from build123d import *

# Parameters (mm, degrees)
SKETCH1_R           = 4
SKETCH1_R_2         = 12
BOSS_EXTRUDE1_DEPTH = 5
CUT_EXTRUDE1_REACH  = 55.898
CHAMFER1_SIZE       = 1


with BuildPart() as part:
    # Sketch1 → Boss-Extrude1 (new body)
    with BuildSketch(Plane.XY):
        with BuildLine():
            Line((-40.864864865, 10.298680477), (-8.432432432, 22.469848314))
            ThreePointArc((-8.432432432, 22.469848314), (0, 24), (8.432432432, 22.469848314))
            Line((8.432432432, 22.469848314), (40.864864865, 10.298680477))
            ThreePointArc((40.864864865, 10.298680477), (48, 0), (40.864864865, -10.298680477))
            Line((40.864864865, -10.298680477), (8.432432432, -22.469848314))
            ThreePointArc((8.432432432, -22.469848314), (0, -24), (-8.432432432, -22.469848314))
            Line((-8.432432432, -22.469848314), (-40.864864865, -10.298680477))
            ThreePointArc((-40.864864865, -10.298680477), (-48, 0), (-40.864864865, 10.298680477))
        make_face()
        with Locations((-37, 0)):
            Circle(SKETCH1_R, mode=Mode.SUBTRACT)
        with Locations((37, 0)):
            Circle(SKETCH1_R, mode=Mode.SUBTRACT)
        Circle(SKETCH1_R_2, mode=Mode.SUBTRACT)
    extrude(amount=BOSS_EXTRUDE1_DEPTH)

    # Sketch2 → Cut-Extrude1 (cut, up to next)
    with BuildSketch(Plane.XY.offset(5), mode=Mode.PRIVATE) as cut_extrude1_sk1:
        with BuildLine():
            Line((21.743091746, 12.134165045), (25.1898452, 10.840675422))
            ThreePointArc((25.1898452, 10.840675422), (27.528705446, 8.50299411), (27.308589183, 5.203513849))
            ThreePointArc((27.308589183, 5.203513849), (26, 0), (27.308589183, -5.203513849))
            ThreePointArc((27.308589183, -5.203513849), (27.528705446, -8.50299411), (25.1898452, -10.840675422))
            Line((25.1898452, -10.840675422), (21.743091746, -12.134165045))
            ThreePointArc((21.743091746, -12.134165045), (17.464066334, -11.171690651), (16.639925188, -6.863882994))
            ThreePointArc((16.639925188, -6.863882994), (18, 0), (16.639925188, 6.863882994))
            ThreePointArc((16.639925188, 6.863882994), (17.464066334, 11.171690651), (21.743091746, 12.134165045))
        make_face()
    cut_extrude1_tool1 = extrude(cut_extrude1_sk1.sketch, amount=-CUT_EXTRUDE1_REACH, mode=Mode.PRIVATE) & part.part
    # Sketch2 → Cut-Extrude1 (cut, up to next)
    with BuildSketch(Plane.XY.offset(5), mode=Mode.PRIVATE) as cut_extrude1_sk2:
        with BuildLine():
            Line((-21.743091746, -12.134165045), (-25.1898452, -10.840675422))
            ThreePointArc((-25.1898452, -10.840675422), (-27.528705446, -8.50299411), (-27.308589183, -5.203513849))
            ThreePointArc((-27.308589183, -5.203513849), (-26, 0), (-27.308589183, 5.203513849))
            ThreePointArc((-27.308589183, 5.203513849), (-27.528705446, 8.50299411), (-25.1898452, 10.840675422))
            Line((-25.1898452, 10.840675422), (-21.743091746, 12.134165045))
            ThreePointArc((-21.743091746, 12.134165045), (-17.464066334, 11.171690651), (-16.639925188, 6.863882994))
            ThreePointArc((-16.639925188, 6.863882994), (-18, 0), (-16.639925188, -6.863882994))
            ThreePointArc((-16.639925188, -6.863882994), (-17.464066334, -11.171690651), (-21.743091746, -12.134165045))
        make_face()
    cut_extrude1_tool2 = extrude(cut_extrude1_sk2.sketch, amount=-CUT_EXTRUDE1_REACH, mode=Mode.PRIVATE) & part.part
    add(cut_extrude1_tool1.solids().sort_by_distance((21.936549, 0, 5))[0], mode=Mode.SUBTRACT)
    add(cut_extrude1_tool2.solids().sort_by_distance((-21.936549, 0, 5))[0], mode=Mode.SUBTRACT)

    # Chamfer1
    chamfer1_edges = [part.edges().sort_by_distance(p)[0] for p in [
        (33, 0, 5),
        (-41, 0, 5),
    ]]
    chamfer(chamfer1_edges, length=CHAMFER1_SIZE)


solid = part.part
Read the model definition and answer for the solid it produces. Units are mm, in the model's axes. A direction names the side the tool comes from. Give positions to 0.01 mm unless a question says otherwise; leave off trailing zeros. Write each loop counter-clockwise with the first axis right and the second up, starting at its lowest first coordinate (ties: lowest second). Pieces come first, ordered by that corner, then holes. Notation, with made-up numbers: (89, 0) -> (115, 0) arc R24 cw to (115, 10) -> close; hole circle Ø10 at (14, 22.25). An arc over 180 degrees is marked (long way). Answer as a JSON object with one key per item and string values. Group by question number.
1) A tool of negligible diameter and unlimited length cuts with its end or side. For faces 4 (the cylindrical face through (-48, 0, 2)), 5 (the cylindrical face through (-26, 0, 3)), from which of +Z, -Z, +X, -X, +Y, -Y can it reach the whole face along a straight path? Write none if from no direction.
2) Find section C-C (z = 1.05). Write down the section's boundary in (x, y), and give its area (3 significant figures).
3) The mould has two halves that part along X. Classify faces 1 (the flat face through (23.49, -11.48, 2.54)), 2 (the flat face through (11.3, -5, 0)), 3 (the cylindrical face through (48, 0, 2)): +X half, -X half, draft (parallel to the pull), parting line (faces both ways), or undercut.
4) Find section A-A (y = 0). Write down the section's boundary in (x, z).
5) Find section D-D (x = 37). Write down the section's boundary in (y, z).
6) Find section B-B (x = 0). Write down the section's boundary in (y, z), and give its area (3 significant figures).
7) Consider L1, parallel to X at y = 7, z = 3.5; L2, parallel to X at y = 1, z = 2.4; L3, parallel to X at y = -10, z = 1.3. Determine where each line is inside the solid, lowest interval first. Write a range as from..to.
8) Each of these flat-tipped pins is pushed along its axis until it touches: P1, Ø3, axis at y = -8, z = 2.5, coming from the +X side; P2, Ø10, axis at x = -3, y = -5, coming from the +Z side; P3, Ø13, axis at x = -37, y = 0, coming from the -Z side; P4, Ø3, axis at x = -13.5, z = 3, coming from the -Y side. Where does it stop, or does it pass through?
Values follow:
{
 "1": {"face 4": "+Z, -Z, -X", "face 5": "+Z, -Z"},
 "2": {"outline": "(-40.86, -10.3) -> (-8.43, -22.47) arc R24 ccw to (8.43, -22.47) -> (40.86, -10.3) arc R11 ccw to (40.86, 10.3) -> (8.43, 22.47) arc R24 ccw to (-8.43, 22.47) -> (-40.86, 10.3) arc R11 ccw to start; hole circle Ø8 at (-37, 0); hole (-27.31, -5.2) arc R4 ccw to (-25.19, -10.84) -> (-21.74, -12.13) arc R4 ccw to (-16.64, -6.86) arc R18 cw to (-16.64, 6.86) arc R4 ccw to (-21.74, 12.13) -> (-25.19, 10.84) arc R4 ccw to (-27.31, 5.2) arc R11 cw to start; hole circle Ø24 at (0, 0); hole (16.64, -6.86) arc R4 ccw to (21.74, -12.13) -> (25.19, -10.84) arc R4 ccw to (27.31, -5.2) arc R11 cw to (27.31, 5.2) arc R4 ccw to (25.19, 10.84) -> (21.74, 12.13) arc R4 ccw to (16.64, 6.86) arc R18 cw to start; hole circle Ø8 at (37, 0)", "area": "2,130 mm2"},
 "3": {"face 1": "undercut", "face 2": "draft", "face 3": "+X half"},
 "4": {"outline": "(-48, 0) -> (-41, 0) -> (-41, 4) -> (-42, 5) -> (-48, 5) -> close; (-33, 0) -> (-26, 0) -> (-26, 5) -> (-32, 5) -> (-33, 4) -> close; (-18, 0) -> (-12, 0) -> (-12, 5) -> (-18, 5) -> close; (12, 0) -> (18, 0) -> (18, 5) -> (12, 5) -> close; (26, 0) -> (33, 0) -> (33, 4) -> (32, 5) -> (26, 5) -> close; (41, 0) -> (48, 0) -> (48, 5) -> (42, 5) -> (41, 4) -> close"},
 "5": {"outline": "(-11.75, 0) -> (-4, 0) -> (-4, 4) -> (-5, 5) -> (-11.75, 5) -> close; (4, 0) -> (11.75, 0) -> (11.75, 5) -> (5, 5) -> (4, 4) -> close"},
 "6": {"outline": "(-24, 0) -> (-12, 0) -> (-12, 5) -> (-24, 5) -> close; (12, 0) -> (24, 0) -> (24, 5) -> (12, 5) -> close", "area": "120 mm2"},
 "7": {"L1": "x = -45.49..-27.78, -16.59..-9.75, 9.75..16.59, 27.78..45.49", "L2": "x = -47.95..-40.87, -33.13..-26.05, -17.97..-11.96, 11.96..17.97, 26.05..33.13, 40.87..47.95", "L3": "x = -41.58..-26.53, -16.68..-6.63, 6.63..16.68, 26.53..41.58"},
 "8": {"P1": "stops at x = 45.87", "P2": "passes through", "P3": "stops at z = 0", "P4": "stops at y = -21.13"}
}
